Geometry check sheet. Reference: the model listing, model coordinates, mm. A direction names the side the tool comes from. Give positions to 0.01 mm unless a question says otherwise; leave off trailing zeros. Loops run counter-clockwise (first coordinate to the right, second up) from the corner with the lowest first, then second, coordinate; pieces in that order, holes last. Notation, with made-up numbers: (-1.75, 48.5) - (52.25, 48.5) arc R18 cw to (52.25, 74.5) - close; hole circle Ø2 at (-22.5, 56). An arc over 180 degrees is marked (long way). Use a Markdown table: item, result. Add a question column.
1. Cross-section at B-B on x = -110. Enter the section's corners in (y, z).
2. Cross-section at D-D on y = 6. Enter the section's corners in (x, z), and give its area (3 significant figures).
3. Material ranges on L1, parallel to X at y = 32, z = 5.75; L2, parallel to X at y = 21, z = 5.75; L3, parallel to X at y = 35.5, z = 1.5, recorded low to high.
4. Cross-section at A-A on y = 32.25. Enter the section's corners in (x, z).
5. Cross-section at C-C on z = 2.75. Enter the section's corners in (x, y).
6. Draft check along X on faces 1 (the flat face through (-4, 27.5, 4)), 2 (the cylindrical face through (-19.19, 31.34, 4.06)), 3 (the cylindrical face through (-121.36, 13.073, 3.944)). Enter one of: pulls with the +X half, pulls with the -X half, needs draft (parallel to the pull), parting line crosses it, or undercut.
7. Depth check by flat-ended pin: P1, Ø2.5, axis at x = -18, y = 12.75, coming from the -Z side; P2, Ø1, axis at y = 9, z = 4, coming from the +X side; P3, Ø2, axis at y = 26.5, z = 3, coming from the -X side. Enter the tip coordinate at first touch or a pass-through.
8. Set-up check for faces 4 (the flat face through (-8, 32, 4)), 5 (the flat face through (-63, 23, 0)): record each of +Z, -Z, +X, -X, +Y, -Y from which the full face is reachable in a straight line by a thin tool's end or side.
from build123d import *

# Parameters (mm, degrees)
BOSS_EXTRUDE1_DEPTH = 8
CHAMFER1_SIZE       = 10
CHAMFER1_SIZE2      = 65
CHAMFER2_SIZE       = 65
CHAMFER2_SIZE2      = 10
FILLET2_R           = 15
FILLET3_R           = 50
SKETCH2_R           = 4
CUT_EXTRUDE1_DEPTH  = 80
SKETCH4_R           = 1.5
CUT_EXTRUDE3_DEPTH  = 15


with BuildPart() as part:
    # Sketch1 → Boss-Extrude1 (new body)
    with BuildSketch(Plane.XY):
        Polygon((0, 17.5), (0, 27.5), (-8, 27.5), (-8, 37), (0, 37), (0, 45), (-125, 45), (-125, 22.5), (-125, 0), (0, 0), (0, 8), (-8, 8), (-8, 17.5), align=None)
    extrude(amount=BOSS_EXTRUDE1_DEPTH)

    # Chamfer1
    chamfer1_edges = [part.edges().sort_by_distance(p)[0] for p in [
        (-125, 0, 4),
    ]]
    chamfer1_side = [part.faces().sort_by_distance(p)[0] for p in [
        (-125, 22.5, 4),
    ]]
    chamfer(chamfer1_edges, length=CHAMFER1_SIZE, length2=CHAMFER1_SIZE2, reference=chamfer1_side[0])

    # Chamfer2
    chamfer2_edges = [part.edges().sort_by_distance(p)[0] for p in [
        (-125, 45, 4),
    ]]
    chamfer2_side = [part.faces().sort_by_distance(p)[0] for p in [
        (-62.5, 45, 4),
    ]]
    chamfer(chamfer2_edges, length=CHAMFER2_SIZE, length2=CHAMFER2_SIZE2, reference=chamfer2_side[0])

    # Fillet2
    # the kernel refuses this fillet: 15 mm, written as the material it takes off along each edge
    with BuildSketch(Plane(origin=(-125, 10, -32.171960879), x_dir=(0, 1, 0), z_dir=(0, 0, 1))) as fillet2_piece_1:
        with BuildLine():
            CenterArc((FILLET2_R * 0.857918956767, -FILLET2_R), FILLET2_R, 90, 81.253837737)
            Line((-FILLET2_R * 0.130452740884, -FILLET2_R * 0.847942815746), (0, 0))
            Line((0, 0), (FILLET2_R * 0.857918956767, 0))
        make_face()
    extrude(amount=72.343921757, mode=Mode.SUBTRACT)
    with BuildSketch(Plane(origin=(-125, 35, -32.171960879), x_dir=(0, -1, 0), z_dir=(0, 0, 1))) as fillet2_piece_2:
        with BuildLine():
            CenterArc((FILLET2_R * 0.857918956767, FILLET2_R), FILLET2_R, 188.746162263, 81.253837737)
            Line((-FILLET2_R * 0.130452740884, FILLET2_R * 0.847942815746), (0, 0))
            Line((0, 0), (FILLET2_R * 0.857918956767, 0))
        make_face()
    extrude(amount=72.343921757, mode=Mode.SUBTRACT)

    # Fillet3
    fillet3_edges = [part.edges().sort_by_distance(p)[0] for p in [
        (-60, 0, 4),
        (-60, 45, 4),
    ]]
    fillet(fillet3_edges, radius=FILLET3_R)

    # Sketch2 → Cut-Extrude1 (cut)
    with BuildSketch(Plane.XY.offset(8)):
        with Locations((-110, 22.868784351)):
            Circle(SKETCH2_R)
    extrude(amount=-CUT_EXTRUDE1_DEPTH, mode=Mode.SUBTRACT)

    # Sketch4 → Cut-Extrude3 (cut)
    with BuildSketch(Plane.XY.offset(8)):
        with Locations((-18, 32.25)):
            Circle(SKETCH4_R)
        with Locations((-18, 12.75)):
            Circle(SKETCH4_R)
    extrude(amount=-CUT_EXTRUDE3_DEPTH, mode=Mode.SUBTRACT)


solid = part.part
Values found:
| question | item | result |
|---|---|---|
| 1 | outline | (7.69, 0) - (18.87, 0) - (18.87, 8) - (7.69, 8) - close; (26.87, 0) - (37.31, 0) - (37.31, 8) - (26.87, 8) - close |
| 2 | outline | (-99, 0) - (0, 0) - (0, 8) - (-99, 8) - close |
| 2 | area | 792 mm2 |
| 3 | L1 | x = -121.3 to -19.48, -16.52 to -8 |
| 3 | L2 | x = -124.88 to -113.54, -106.46 to 0 |
| 3 | L3 | x = -116.8 to -8 |
| 4 | outline | (-121.07, 0) - (-19.5, 0) - (-19.5, 8) - (-121.07, 8) - close; (-16.5, 0) - (-8, 0) - (-8, 8) - (-16.5, 8) - close |
| 5 | outline | (-125, 22.5) arc R15 ccw to (-112.28, 8.04) - (-63.78, 0.58) arc R50 ccw to (-56.18, 0) - (0, 0) - (0, 8) - (-8, 8) - (-8, 17.5) - (0, 17.5) - (0, 27.5) - (-8, 27.5) - (-8, 37) - (0, 37) - (0, 45) - (-56.18, 45) arc R50 ccw to (-63.78, 44.42) - (-112.28, 36.96) arc R15 ccw to start; hole circle Ø8 at (-110, 22.87); hole circle Ø3 at (-18, 12.75); hole circle Ø3 at (-18, 32.25) |
| 6 | face 1 | needs draft |
| 6 | face 2 | undercut |
| 6 | face 3 | pulls with the -X half |
| 7 | P1 | passes through |
| 7 | P2 | stops at x = -8 |
| 7 | P3 | stops at x = -124.62 |
| 8 | face 4 | +Z, -Z, +X |
| 8 | face 5 | -Z, +X, -X, +Y, -Y |
